Autodesk Inventor part; units mm, degrees
ref_plane "YZ Plane" through (0, 0, 0) normal (1, 0, 0) x (0, 1, 0)
ref_plane "XZ Plane" through (0, 0, 0) normal (0, 1, 0) x (-1, 0, 0)
ref_plane "XY Plane" through (0, 0, 0) normal (0, 0, 1) x (1, 0, 0)
sketch "Sketch1" plane through (0, 0, 0) normal (0, 1, 0) x (-1, 0, 0)
  circle A0 centre (0, 0) radius 100
  dimension "d0" = 200
extrude "Extrusion1" add sketch "Sketch1" along normal blind 4
sketch "Sketch2" plane through (0, 4, 0) normal (0, 1, 0) x (1, 0, 0)
  circle A0 centre (0, 0) radius 100
  circle A1 centre (0, 0) radius 5
  dimension "d3" = 10
hole "Hole1" at (0, 4, 0) direction (0, -1, 0) diameter 11 end through all
sketch "Sketch4" plane through (0, 4, 0) normal (0, 1, 0) x (1, 0, 0)
  circle A0 centre (0, 57) radius 3.175
  circle A1 centre (-51.9615, -30) radius 3.175
  circle A2 centre (49.3634, -28.5) radius 3.175
  circle A3 centre (0, 0) radius 100
  line L0 (0, 0) -> (0, 57) construction
  line L1 (0, 0) -> (49.3634, -28.5) construction
  line L2 (0, 0) -> (57, 0) construction
  line L3 (0, 0) -> (-51.9615, -30) construction
  line L4 (0, 0) -> (60, 0) construction
  dimension "d28" = 360
  dimension "d24" = 6.35
  dimension "d37" = 57
  dimension "d38" = 57
  dimension "d39" = 30
  dimension "d40" = 60
  dimension "d41" = 150
hole "Hole3" at (0, 4, -57) at (49.3634, 4, 28.5) at (-51.9615, 4, 30) direction (0, -1, 0) diameter 6.6 end through all
properties part number "bpPlate" material "Steel"
Here's how the part is built. I have some questions about the finished solid (model axes, mm). Coordinates: 2 decimals unless noted, no trailing zeros. Order: outer loops, then holes, each group sorted by start corner. A loop starts at its lowest first (then second) coordinate and runs counter-clockwise, first axis right, second up. Notation, with made-up numbers: M 42,89.25 L 52,89.25 A9 cw 52,102.25 Z; hole C 79.25,-30 d4. An arc over 180 degrees is marked long. Answer as a JSON object with one key per item and string values. Group by question number.
(1) Suppose I cut it at C-C, the plane y = 1. Please give me the cut outline in (x, z), then the cut area to 3 significant figures.
(2) Suppose I cut it at A-A, the plane x = 0. Please give me the cut outline in (y, z), then the cut area to 3 significant figures.
(3) Suppose I cut it at D-D, the plane z = -57. Please give me the cut outline in (x, y), then the cut area to 3 significant figures.
(4) Suppose I cut it at B-B, the plane z = 0. Please give me the cut outline in (x, y), then the cut area to 3 significant figures.
(5) I need wall thicknesses on probe 1 along Z at (x, y) = (0, 2.1); probe 2 along X at (y, z) = (2.5, 28.5); probe 3 along X at (y, z) = (1.25, -56). Which ranges of each line are inside material? Lowest first, please.
(6) For pin 1 (12.5 mm diameter, centred on x = 0, z = 0, fed in from -Y); pin 2 (1.5 mm diameter, centred on x = -24, y = 2.5, fed in from +Z); pin 3 (4 mm diameter, centred on x = 0, z = -57, fed in from +Y) (3 decimals); pin 4 (1.5 mm diameter, centred on y = 3, z = -45, fed in from -X), each with a flat end and sliding along its axis, tell me the tip position at first contact or that it passes through.
(7) If we mould it in two halves opening along Z, with no side actions, what happens to faces 1 (the face through (-95.38, 1.97, -30.04)), 2 (the face through (1, 4, -21)), 3 (the face through (-49.034, 1.972, 31.523))? For each: released by +Z, released by -Z, zero draft, split by the parting line, or undercut.
Values found:
{
 "1": {"outline": "C 0,0 d200; hole C -51.96,30 d6.6; hole C 0,0 d11; hole C 0,-57 d6.6; hole C 49.36,28.5 d6.6", "area": "31,200 mm^2"},
 "2": {"outline": "M 0,-100 L 4,-100 L 4,-60.3 L 0,-60.3 Z; M 0,-53.7 L 4,-53.7 L 4,-5.5 L 0,-5.5 Z; M 0,5.5 L 4,5.5 L 4,100 L 0,100 Z", "area": "730 mm^2"},
 "3": {"outline": "M -82.16,0 L -3.3,0 L -3.3,4 L -82.16,4 Z; M 3.3,0 L 82.16,0 L 82.16,4 L 3.3,4 Z", "area": "631 mm^2"},
 "4": {"outline": "M -100,0 L -5.5,0 L -5.5,4 L -100,4 Z; M 5.5,0 L 100,0 L 100,4 L 5.5,4 Z", "area": "756 mm^2"},
 "5": {"probe 1": "z = -100 to -60.3, -53.7 to -5.5, 5.5 to 100", "probe 2": "x = -95.85 to -54.9, -49.02 to 46.06, 52.66 to 95.85", "probe 3": "x = -82.85 to -3.14, 3.14 to 82.85"},
 "6": {"pin 1": "stops at y = 0", "pin 2": "stops at z = 97.26", "pin 3": "passes through", "pin 4": "stops at x = -89.68"},
 "7": {"face 1": "split by the parting line", "face 2": "zero draft", "face 3": "undercut"}
}
